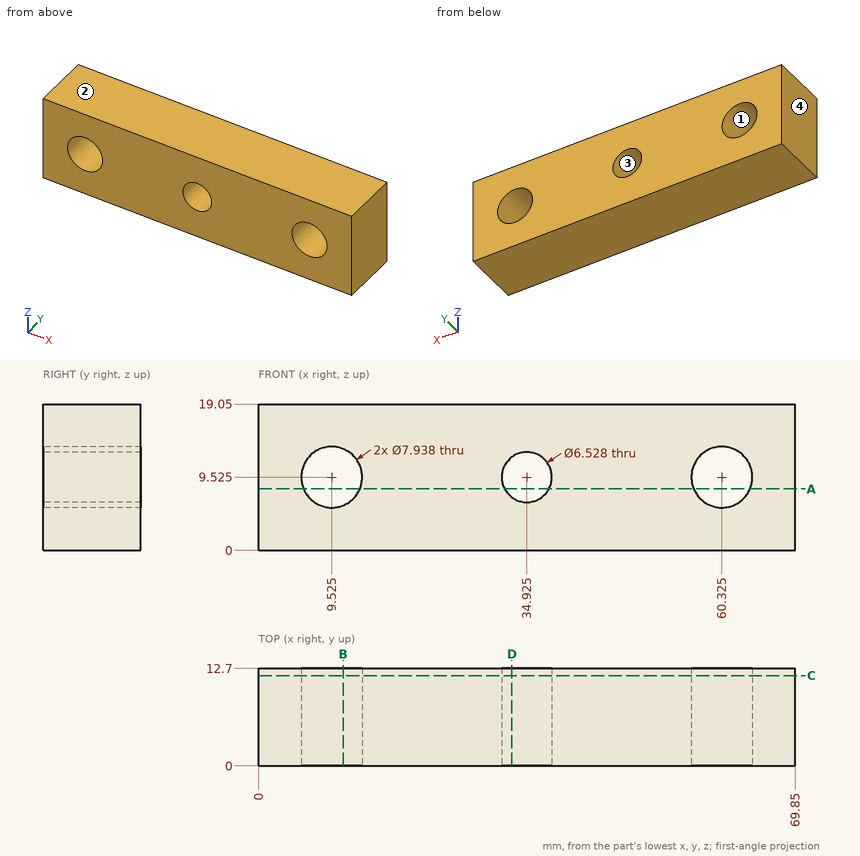
Study the drawing (mm; zero at the part's minimum x, y, z) and answer. Give positions to 0.01 mm unless a question says otherwise; leave off trailing zeros. Write each loop counter-clockwise with the first axis right and the second up, starting at its lowest first coordinate (ties: lowest second). Pieces come first, ordered by that corner, then holes.
Item 1: Determine the mould class of the marked faces 1, 2, 3 and 4 for opening direction X: released by +X, released by -X, zero draft, split by the parting line, or undercut.
Item 2: Section C-C, the plane y = 11.75 is taken. Count the separate pieces of the cut face and the enclosed holes in it, plus the area to 3 significant figures.
Item 3: Section B-B, the plane x = 11 is taken. Write down the section's boundary in (y, z), plus the area to 3 significant figures.
Item 4: Section A-A, the plane z = 8 is taken. Write down the section's boundary in (x, y).
Item 5: Section D-D, the plane x = 33 is taken. Write down the section's boundary in (y, z), plus the area to 3 significant figures.
Item 6: Find the intervals of material crossed by line 1 along X through (y, z) = (3.5, 9); line 2 along Z through (x, y) = (9, 11.75); line 3 along Z through (x, y) = (8, 5), in increasing order.
Completed:
1. face 1: undercut
1. face 2: zero draft
1. face 3: undercut
1. face 4: released by -X
2. separate pieces: 1
2. enclosed holes: 3
2. area: 1,200 mm2
3. outline: (0, 0) - (12.7, 0) - (12.7, 5.84) - (0, 5.84) - close; (0, 13.21) - (12.7, 13.21) - (12.7, 19.05) - (0, 19.05) - close
3. area: 148 mm2
4. outline: (0, 0) - (5.86, 0) - (5.86, 12.7) - (0, 12.7) - close; (13.19, 0) - (32.04, 0) - (32.04, 12.7) - (13.19, 12.7) - close; (37.81, 0) - (56.66, 0) - (56.66, 12.7) - (37.81, 12.7) - close; (63.99, 0) - (69.85, 0) - (69.85, 12.7) - (63.99, 12.7) - close
5. outline: (0, 0) - (12.7, 0) - (12.7, 6.89) - (0, 6.89) - close; (0, 12.16) - (12.7, 12.16) - (12.7, 19.05) - (0, 19.05) - close
5. area: 175 mm2
6. line 1: x = 0 to 5.59, 13.46 to 31.7, 38.15 to 56.39, 64.26 to 69.85
6. line 2: z = 0 to 5.59, 13.46 to 19.05
6. line 3: z = 0 to 5.86, 13.19 to 19.05
